from build123d import *

# Parameters (mm, degrees)
SKETCH_1_R      = 1.6
EXTRUDE_1_DEPTH = 3
FILLET_1_R      = 2
FILLET_2_R      = 10


with BuildPart() as part:
    # 草图1 → 凸台-拉伸1 (new body)
    with BuildSketch(Plane.XY):
        Polygon((0, 0), (6, 0), (6, 36), (45, 36), (45, 42), (6, 42), (6, 75), (0, 75), (0, 42), (-39, 42), (-39, 36), (0, 36), align=None)
        with Locations((40, 39)):
            Circle(SKETCH_1_R, mode=Mode.SUBTRACT)
        with Locations((-34, 39)):
            Circle(SKETCH_1_R, mode=Mode.SUBTRACT)
        with Locations((3, 7.5)):
            Circle(SKETCH_1_R, mode=Mode.SUBTRACT)
        with Locations((3, 70.5)):
            Circle(SKETCH_1_R, mode=Mode.SUBTRACT)
        Polygon((3, 43.306086205), (-2.288898942, 39.401411526), (3, 34.92685231), (8.288898942, 39.401411526), align=None, mode=Mode.SUBTRACT)
    extrude(amount=EXTRUDE_1_DEPTH)

    # 圆角1
    fillet_1_edges = [part.edges().sort_by_distance(p)[0] for p in [
        (-39, 36, 1.5),
        (-39, 42, 1.5),
        (0, 75, 1.5),
        (6, 75, 1.5),
        (45, 42, 1.5),
        (45, 36, 1.5),
        (6, 0, 1.5),
        (0, 0, 1.5),
    ]]
    fillet(fillet_1_edges, radius=FILLET_1_R)

    # 圆角2
    fillet_2_edges = [part.edges().sort_by_distance(p)[0] for p in [
        (0, 36, 1.5),
        (0, 42, 1.5),
        (6, 42, 1.5),
        (6, 36, 1.5),
    ]]
    fillet(fillet_2_edges, radius=FILLET_2_R)


solid = part.part
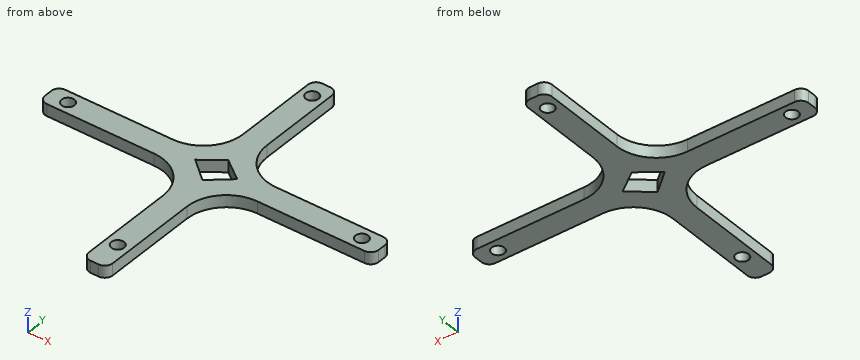
Verification items for the finished model (mm, model axes). Give positions to 0.01 mm unless a question says otherwise; leave off trailing zeros. Write each loop counter-clockwise with the first axis right and the second up, starting at its lowest first coordinate (ties: lowest second). Pieces come first, ordered by that corner, then holes.
(1) Cross-section at B-B (y = 7.5). Enter the section's corners in (x, z), plus the area to 3 significant figures.
(2) Material ranges on line 1 (Y direction, x = 3, z = 1.3); line 2 (Y direction, x = 40, z = 1.8); line 3 (Y direction, x = 17.5, z = 2.7), recorded low to high.
(3) Cross-section at D-D (y = 32). Enter the section's corners in (x, z), plus the area to 3 significant figures.
(4) Gauge pin test, flat ends, axial feed: pin 1 (1 mm diameter, centred on x = 23, z = 2.5, fed in from -Y); pin 2 (4 mm diameter, centred on x = 3, y = 7.5, fed in from +Z); pin 3 (1.5 mm diameter, centred on y = 14, z = 1, fed in from +X); pin 4 (1.5 mm diameter, centred on y = 64.5, z = 1.5, fed in from -X). Record the tip position at first contact, or that the pin passes through.
(5) Cross-section at A-A (x = 40). Enter the section's corners in (y, z), plus the area to 3 significant figures.
(6) Cross-section at C-C (z = 1.25). State how many separate pieces and enclosed holes the cut face has, plus the area to 3 significant figures.
Worked out:
1. outline: (0, 0) - (1.4, 0) - (1.4, 3) - (0, 3) - close; (4.6, 0) - (6, 0) - (6, 3) - (4.6, 3) - close
1. area: 8.40 mm2
2. line 1: y = 0 to 5.9, 9.1 to 34.93, 43.31 to 68.9, 72.1 to 75
2. line 2: y = 36 to 37.4, 40.6 to 42
2. line 3: y = 36 to 42
3. outline: (-2, 0) - (8, 0) - (8, 3) - (-2, 3) - close
3. area: 30.0 mm2
4. pin 1: stops at y = 36
4. pin 2: stops at z = 3
4. pin 3: stops at x = 6
4. pin 4: stops at x = 0
5. outline: (36, 0) - (37.4, 0) - (37.4, 3) - (36, 3) - close; (40.6, 0) - (42, 0) - (42, 3) - (40.6, 3) - close
5. area: 8.40 mm2
6. separate pieces: 1
6. enclosed holes: 5
6. area: 920 mm2
